```python
from build123d import *

# Parameters (mm, degrees)
BOSS_EXTRUDE1_DEPTH = 30
FILLET1_R           = 85
FILLET2_R           = 4


with BuildPart() as part:
    # Sketch1 → Boss-Extrude1 (new body)
    with BuildSketch(Plane(origin=(0, 0, 0), x_dir=(1, 0, 0), z_dir=(0, 1, 0))):
        with BuildLine():
            Line((-12, -21), (-12, -15.5))
            Line((-12, -15.5), (-14, -15.5))
            ThreePointArc((-14, -15.5), (-16.560660172, -16.560660172), (-15.5, -14))
            Line((-15.5, -14), (-15.5, 14))
            ThreePointArc((-15.5, 14), (-16.560660172, 16.560660172), (-14, 15.5))
            Line((-14, 15.5), (14, 15.5))
            ThreePointArc((14, 15.5), (15.5, 17), (17, 15.5))
            ThreePointArc((17, 15.5), (16.560660172, 14.439339828), (15.5, 14))
            Line((15.5, 14), (15.5, -14))
            ThreePointArc((15.5, -14), (16.560660172, -14.439339828), (17, -15.5))
            ThreePointArc((17, -15.5), (15.5, -17), (14, -15.5))
            Line((14, -15.5), (12, -15.5))
            Line((12, -15.5), (12, -21))
            Line((12, -21), (21, -21))
            Line((21, -21), (21, 21))
            Line((21, 21), (-21, 21))
            Line((-21, 21), (-21, -21))
            Line((-21, -21), (-12, -21))
        make_face()
        with BuildLine():
            Line((-12, -15.5), (-12, -3.5))
            ThreePointArc((-12, -3.5), (-1.767766953, 12.374368671), (12.5, 0))
            ThreePointArc((12.5, 0), (12.374368671, -1.767766953), (12, -3.5))
            Line((12, -3.5), (12, -15.5))
            Line((12, -15.5), (14, -15.5))
            ThreePointArc((14, -15.5), (14.439339828, -14.439339828), (15.5, -14))
            Line((15.5, -14), (15.5, 14))
            ThreePointArc((15.5, 14), (14.439339828, 14.439339828), (14, 15.5))
            Line((14, 15.5), (-14, 15.5))
            ThreePointArc((-14, 15.5), (-14.439339828, 14.439339828), (-15.5, 14))
            Line((-15.5, 14), (-15.5, -14))
            ThreePointArc((-15.5, -14), (-14.439339828, -14.439339828), (-14, -15.5))
            Line((-14, -15.5), (-12, -15.5))
        make_face()
    extrude(amount=BOSS_EXTRUDE1_DEPTH)

    # Fillet1
    fillet1_edges = [part.edges().sort_by_distance(p)[0] for p in [
        (-12, 15, 3.5),
        (12, 15, 3.5),
    ]]
    fillet(fillet1_edges, radius=FILLET1_R)

    # Fillet2
    fillet2_edges = [part.edges().sort_by_distance(p)[0] for p in [
        (-12, 15, 21),
        (-21, 15, 21),
        (-21, 15, -21),
        (21, 15, -21),
        (21, 15, 21),
        (12, 15, 21),
    ]]
    fillet(fillet2_edges, radius=FILLET2_R)


solid = part.part
```
Here's how the part is built. I have some questions about the finished solid (model axes, mm). A direction names the side the tool comes from. Round coordinates to 2 decimals unless told otherwise and drop trailing zeros. Loops run counter-clockwise (first coordinate to the right, second up) from the corner with the lowest first, then second, coordinate; pieces in that order, holes last.
1. Suppose I cut it at A-A, the plane y = 16. Please give me the cut outline in (x, z), and give its area (3 significant figures).
Answers:
outline: (-21, -17) arc R4 ccw to (-17, -21) - (17, -21) arc R4 ccw to (21, -17) - (21, 17) arc R4 ccw to (17, 21) - (16, 21) arc R4 ccw to (12, 17) - (12, 9.86) arc R85 ccw to (12.44, 1.26) arc R12.5 cw (long way) to (-12.44, 1.26) arc R85 ccw to (-12, 9.86) - (-12, 17) arc R4 ccw to (-16, 21) - (-17, 21) arc R4 ccw to (-21, 17) - close; hole circle Ø3 at (-15.5, -15.5); hole circle Ø3 at (-15.5, 15.5); hole circle Ø3 at (15.5, -15.5); hole circle Ø3 at (15.5, 15.5)
area: 962 mm2
2. Will these pins go through, and if not, where does the flat tip stop? pin 1 (6 mm diameter, centred on x = -16.5, z = -6.5, fed in from -Y); pin 2 (10 mm diameter, centred on x = -8.5, y = 10.5, fed in from +Z).
Answers:
pin 1: stops at y = 0
pin 2: stops at z = 20.12
3. Suppose I cut it at C-C, the plane z = -6. Please give me the cut outline in (x, y), and give its area (3 significant figures).
Answers:
outline: (-21, 0) - (-10.97, 0) - (-10.97, 30) - (-21, 30) - close; (10.97, 0) - (21, 0) - (21, 30) - (10.97, 30) - close
area: 602 mm2
4. If I drill on probe 1 along X at (y, z) = (10.25, -15.5); probe 2 along X at (y, z) = (8.75, 15.5); probe 3 along X at (y, z) = (26, 9), over which ranges is the centre line in solid material (lowest first)?
Answers:
probe 1: x = -21 to -17, -14 to 14, 17 to 21
probe 2: x = -21 to -17, -14 to -12, 12 to 14, 17 to 21
probe 3: x = -21 to -12, 12 to 21
5. For faces 5 (the face through (12, 15, 13)), 6 (the face through (16.5, 14.8, 21)), which set-ups out of +Z, -Z, +X, -X, +Y, -Y let a thin tool reach every point of the face, with its end or its side?
Answers:
face 5: +Z, +Y, -Y
face 6: +Z, +X, -X, +Y, -Y
6. Suppose I cut it at B-B, the plane z = 5. Please give me the cut outline in (x, y), and give its area (3 significant figures).
Answers:
outline: (-21, 0) - (-12.14, 0) - (-12.14, 30) - (-21, 30) - close; (12.14, 0) - (21, 0) - (21, 30) - (12.14, 30) - close
area: 532 mm2
7. Thinking about a two-plate mould opening in Z: for faces 1 (the face through (12.11, 15.21, 5.5)), 2 (the face through (-19.859, 15.21, -19.797)), 3 (the face through (-12.106, 15.21, 5.618)), 4 (the face through (13.141, 15.21, 19.797)), which applies, released by +Z, released by -Z, zero draft, split by the parting line, or undercut?
Answers:
face 1: undercut
face 2: released by -Z
face 3: undercut
face 4: released by +Z
8. Suppose I cut it at D-D, the plane x = 0. Please give me the cut outline in (y, z).
Answers:
outline: (0, -21) - (30, -21) - (30, -12.5) - (0, -12.5) - close
